Geometry check sheet. Reference: the model listing, model coordinates, mm. A direction names the side the tool comes from. Round coordinates to 2 decimals unless told otherwise and drop trailing zeros. Loops run counter-clockwise (first coordinate to the right, second up) from the corner with the lowest first, then second, coordinate; pieces in that order, holes last.
```python
from build123d import *

# Parameters (mm, degrees)
SKETCH1_R           = 11
SKETCH1_R_2         = 2
SKETCH1_R_3         = 1.425
BOSS_EXTRUDE1_DEPTH = 2
SKETCH1_3_R         = 5
SKETCH1_3_R_2       = 2
BOSS_EXTRUDE2_DEPTH = 12
CHAMFER1_SIZE       = 0.25


with BuildPart() as part:
    # Sketch1 → Boss-Extrude1 (new body)
    with BuildSketch(Plane(origin=(0, 0, 0), x_dir=(1, 0, 0), z_dir=(0, 1, 0))):
        Circle(SKETCH1_R)
        Circle(SKETCH1_R_2, mode=Mode.SUBTRACT)
        with Locations((-5.5, 5.5)):
            Circle(SKETCH1_R_3, mode=Mode.SUBTRACT)
        with Locations((5.5, 5.5)):
            Circle(SKETCH1_R_3, mode=Mode.SUBTRACT)
        with Locations((5.5, -5.5)):
            Circle(SKETCH1_R_3, mode=Mode.SUBTRACT)
        with Locations((-5.5, -5.5)):
            Circle(SKETCH1_R_3, mode=Mode.SUBTRACT)
    extrude(amount=-BOSS_EXTRUDE1_DEPTH)

    # Sketch1<3> → Boss-Extrude2 (add)
    with BuildSketch(Plane(origin=(0, 0, 0), x_dir=(1, 0, 0), z_dir=(0, 1, 0))):
        Circle(SKETCH1_3_R)
        Circle(SKETCH1_3_R_2, mode=Mode.SUBTRACT)
    extrude(amount=-BOSS_EXTRUDE2_DEPTH)

    # Chamfer1
    chamfer1_edges = [part.edges().sort_by_distance(p)[0] for p in [
        (-5, -12, 0),
        (-5, -2, 0),
        (-2, -12, 0),
        (-11, -2, 0),
        (-11, 0, 0),
    ]]
    chamfer(chamfer1_edges, length=CHAMFER1_SIZE)


solid = part.part
```
1) Sectioned sample at C-C, the plane y = -9. Record the cut outline in (x, z).
Report:
outline: circle Ø10 at (0, 0); hole circle Ø4 at (0, 0)
2) Sectioned sample at B-B, the plane x = 0. Record the cut outline in (y, z).
Report:
outline: (-12, -4.75) - (-11.75, -5) - (-2.25, -5) - (-2, -5.25) - (-2, -10.75) - (-1.75, -11) - (-0.25, -11) - (0, -10.75) - (0, -2) - (-11.75, -2) - (-12, -2.25) - close; (-12, 2.25) - (-11.75, 2) - (0, 2) - (0, 10.75) - (-0.25, 11) - (-1.75, 11) - (-2, 10.75) - (-2, 5.25) - (-2.25, 5) - (-11.75, 5) - (-12, 4.75) - close
3) Access from +Z, -Z, +X, -X, +Y, -Y to the whole of each face (thin tool, end or side, straight path). Record for faces 5 (the face through (-1.08, -6.93, 4.88)), 6 (the face through (-6.55, -0.986, -6.463)).
Report:
face 5: -Y
face 6: +Y, -Y
4) Scan lines: line 1 along Z through (x, y) = (-5.5, -1.1) (3 decimals); line 2 along X through (y, z) = (-3.25, 0). Record each from-to range of solid material in increasing order.
Report:
line 1: z = -9.526 to -6.925, -4.075 to 4.075, 6.925 to 9.526
line 2: x = -5 to -2, 2 to 5
5) Sectioned sample at A-A, the plane z = 0. Record the cut outline in (x, y), then the cut area to 3 significant figures.
Report:
outline: (-11, -1.75) - (-10.75, -2) - (-5.25, -2) - (-5, -2.25) - (-5, -11.75) - (-4.75, -12) - (-2.25, -12) - (-2, -11.75) - (-2, 0) - (-10.75, 0) - (-11, -0.25) - close; (2, -11.75) - (2.25, -12) - (4.75, -12) - (5, -11.75) - (5, -2.25) - (5.25, -2) - (10.75, -2) - (11, -1.75) - (11, -0.25) - (10.75, 0) - (2, 0) - close
area: 95.8 mm2
6) Sectioned sample at D-D, the plane z = -6. State how many separate pieces and enclosed holes the cut face has, then the cut area to 3 significant figures.
Report:
separate pieces: 3
enclosed holes: 0
area: 26.1 mm2
7) Mould release check, pull along X, two halves, no side actions. Record for faces 1 (the face through (-2.38, -0.99, 10.74)), 2 (the face through (4.45, -0.986, -6.463)), 3 (the face through (4.45, -0.986, 4.537)), 4 (the face through (5, -2, -3)): +X half, -X half, draft (parallel to the pull), parting line (faces both ways), or undercut.
Report:
face 1: parting line
face 2: undercut
face 3: undercut
face 4: draft
8) Gauge pin test, flat ends, axial feed: pin 1 (3 mm diameter, centred on y = -6.5, z = -2.5, fed in from +X); pin 2 (1 mm diameter, centred on y = -7, z = -6, fed in from +X); pin 3 (1 mm diameter, centred on x = 3, y = -3.5, fed in from +Z); pin 4 (3 mm diameter, centred on x = 4.5, z = 6.5, fed in from -Y). Record the tip position at first contact, or that the pin passes through.
Report:
pin 1: stops at x = 4.9
pin 2: passes through
pin 3: stops at z = 4.33
pin 4: stops at y = -2
